from build123d import *

# Parameters (mm, degrees)
SKETCH1_R           = 4.25
BOSS_EXTRUDE1_DEPTH = 6
SKETCH2_R           = 1.5
CUT_EXTRUDE1_DEPTH  = 413.628161909


with BuildPart() as part:
    # Sketch1 → Boss-Extrude1 (new body)
    with BuildSketch(Plane.XY):
        with BuildLine():
            Line((-384, 99), (-319, 99))
            Line((-319, 99), (-319, 105))
            Line((-319, 105), (-314, 105))
            ThreePointArc((-314, 105), (-306.928932188, 102.071067812), (-304, 95))
            Line((-304, 95), (-304, 30))
            ThreePointArc((-304, 30), (-306.928932188, 22.928932188), (-314, 20))
            Line((-314, 20), (-319, 20))
            Line((-319, 20), (-319, 26))
            Line((-319, 26), (-384, 26))
            Line((-384, 26), (-384, 20))
            Line((-384, 20), (-389, 20))
            ThreePointArc((-389, 20), (-396.071067812, 22.928932188), (-399, 30))
            Line((-399, 30), (-399, 95))
            ThreePointArc((-399, 95), (-396.071067812, 102.071067812), (-389, 105))
            Line((-389, 105), (-384, 105))
            Line((-384, 105), (-384, 99))
        make_face()
        with Locations((-316, 62.5)):
            Circle(SKETCH1_R, mode=Mode.SUBTRACT)
        with Locations(Location((-387, 62.5, 0), (0, 0, 180))):
            Circle(SKETCH1_R, mode=Mode.SUBTRACT)
    extrude(amount=BOSS_EXTRUDE1_DEPTH)

    # Sketch2 → Cut-Extrude1 (cut, through all)
    with BuildSketch(Plane.XY.offset(6)):
        with Locations((-384, 26)):
            Circle(SKETCH2_R)
        with Locations((-319, 26)):
            Circle(SKETCH2_R)
        with Locations((-384, 99)):
            Circle(SKETCH2_R)
        with Locations((-319, 99)):
            Circle(SKETCH2_R)
    extrude(amount=-CUT_EXTRUDE1_DEPTH, mode=Mode.SUBTRACT)


solid = part.part
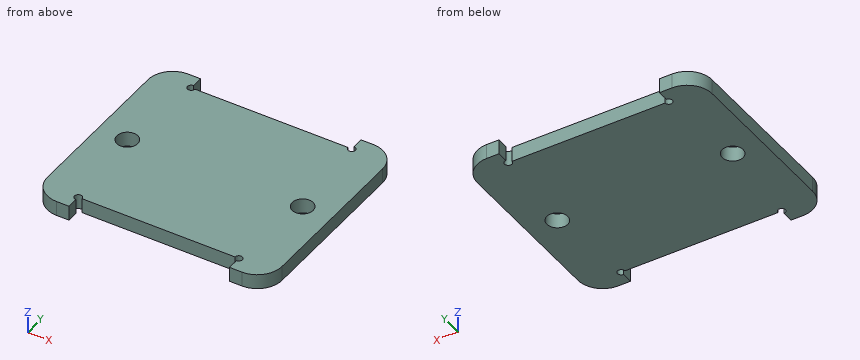
Model file for the job. Use its own axes, mm. Round coordinates to 2 decimals unless told otherwise and drop trailing zeros. Order: outer loops, then holes, each group sorted by start corner. A loop starts at its lowest first (then second) coordinate and runs counter-clockwise, first axis right, second up.
(1) Band-saw the part on A-A (y = 62.5). List the corners of the cut face in (x, z).
(2) Pin check, flat tips, straight feed: pin 1 (2 mm diameter, centred on y = 22, z = 4, fed in from +X); pin 2 (3 mm diameter, centred on x = -361, z = 1.5, fed in from +Y); pin 3 (3 mm diameter, centred on x = -349, z = 4, fed in from -Y). Stop position of each tip, or through.
(3) Drill centre lines: line 1 (X direction, y = 66, z = 2.7); line 2 (Y direction, x = -316, z = 2.2); line 3 (Y direction, x = -325.5, z = 0.4). Where is each one in solid material? Low to high.
(4) Band-saw the part on C-C (x = -352). List the corners of the cut face in (y, z).
(5) Band-saw the part on B-B (z = 1.25). List the corners of the cut face in (x, y).
Verdict:
1. outline: (-399, 0) - (-391.25, 0) - (-391.25, 6) - (-399, 6) - close; (-382.75, 0) - (-320.25, 0) - (-320.25, 6) - (-382.75, 6) - close; (-311.75, 0) - (-304, 0) - (-304, 6) - (-311.75, 6) - close
2. pin 1: stops at x = -306.86
2. pin 2: stops at y = 99
2. pin 3: stops at y = 26
3. line 1: x = -399 to -389.41, -384.59 to -318.41, -313.59 to -304
3. line 2: y = 20 to 58.25, 66.75 to 105
3. line 3: y = 26 to 99
4. outline: (26, 0) - (99, 0) - (99, 6) - (26, 6) - close
5. outline: (-399, 30) arc R10 ccw to (-389, 20) - (-384, 20) - (-384, 24.5) arc R1.5 cw (long way) to (-382.5, 26) - (-320.5, 26) arc R1.5 cw (long way) to (-319, 24.5) - (-319, 20) - (-314, 20) arc R10 ccw to (-304, 30) - (-304, 95) arc R10 ccw to (-314, 105) - (-319, 105) - (-319, 100.5) arc R1.5 cw (long way) to (-320.5, 99) - (-382.5, 99) arc R1.5 cw (long way) to (-384, 100.5) - (-384, 105) - (-389, 105) arc R10 ccw to (-399, 95) - close; hole circle Ø8.5 at (-387, 62.5); hole circle Ø8.5 at (-316, 62.5)
